from build123d import *

# Parameters (mm, degrees)
F0_W     = 152.4
F0_H     = 152.4
F1_DEPTH = 12.7
F2_R     = 50.8
F4_D     = 7.62
F4_DEPTH = 15.24
F4_TIP   = 2.2892789585
F5_R     = 2.54


with BuildPart() as f1:
    # F0 (on Top) → F1 (new body)
    with BuildSketch(Plane.XY):
        with Locations((1.9777435809, -47.0201134945)):
            Rectangle(F0_W, F0_H)
    extrude(amount=F1_DEPTH)

    # F2
    f2_edges = [f1.edges().sort_by_distance(p)[0] for p in [
        (-74.222256, 29.179887, 6.35),
        (78.177744, 29.179887, 6.35),
    ]]
    fillet(f2_edges, radius=F2_R)

    # F4
    with Locations(Plane.XZ.offset(123.2201134945)):
        with Locations((40.0777435809, 6.35), (1.9777435809, 6.35), (-36.1222564191, 6.35)):
            Hole(F4_D / 2, depth=F4_DEPTH)
            with Locations((0, 0, -(F4_DEPTH + F4_TIP / 2))):  # 118° drill point
                Cone(0, F4_D / 2, F4_TIP, mode=Mode.SUBTRACT)

    # F5
    f5_edges = [f1.edges().sort_by_distance(p)[0] for p in [
        (78.177744, -72.420113, 12.7),
        (78.177744, -72.420113, 0),
    ]]
    fillet(f5_edges, radius=F5_R)


solid = f1.part
The listing builds one solid part. Answer for the finished solid, in the listing's coordinates (mm). A direction names the side the tool comes from. Round coordinates to 2 decimals unless told otherwise and drop trailing zeros. Write each question's results on one line, items separated by ' | '. Start each with the question number.
Item 1: The mould has two halves that part along Z. Classify faces 1 (the cylindrical face through (-0.07, -115.493, 9.563)), 2 (the flat face through (1, -47, 12.7)), 3 (the flat face through (78.178, -73, 6)): +Z half, -Z half, draft (parallel to the pull), parting line (faces both ways), or undercut.
Item 2: Given pin 1 Ø6 at (x, z) = (-36.12, 6.35) entering from -Y; pin 2 Ø1 at (x, z) = (30.5, 11) entering from +Y; pin 3 Ø6 at (x, z) = (40.08, 6.35) entering from +Y, each flat-ended and moving along its own axis, determine where each tip first touches the part or whether it passes through.
Item 3: Which of the six approach directions +Z, -Z, +X, -X, +Y, -Y give full straight-line access (tool end or side, diameter ignored) to faces 4 (the cylindrical face through (-32.316, -115.493, 6.518)), 5 (the flat face through (-74.222, -73, 6))?
Item 4: Straight lines are drawn through the part: probe 1 along X at (y, z) = (-114, 6.35); probe 2 along Z at (x, y) = (40, -109); probe 3 along X at (y, z) = (-6, 2). For each, find the intervals that lie inside material, in ascending order.
Answer block:
1) face 1: undercut | face 2: +Z half | face 3: draft
2) pin 1: stops at y = -107.49 | pin 2: stops at y = 29.07 | pin 3: stops at y = 28.24
3) face 4: -Y | face 5: +Z, -Z, -X, +Y, -Y
4) probe 1: x = -74.22 to -39.93, -32.31 to -1.83, 5.79 to 36.27, 43.89 to 78.18 | probe 2: z = 0 to 2.54, 10.16 to 12.7 | probe 3: x = -71.7 to 75.66
